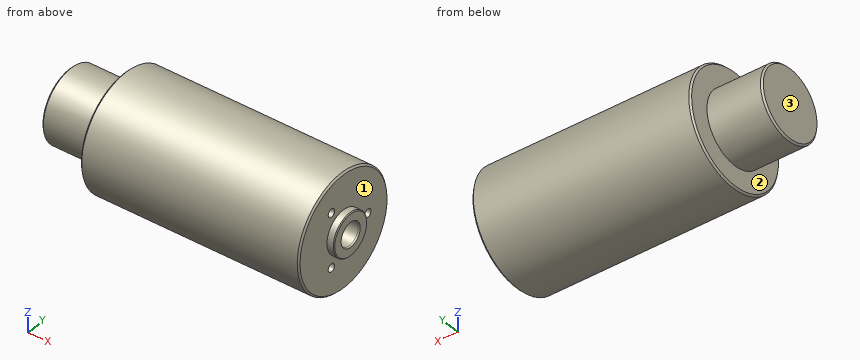
from build123d import *

# Parameters (mm, degrees)
CHANFREIN2_SIZE                   = 0.25
R_P_TITION_CIRCULAIRE1_COUNT      = 3
CHANFREIN3_SIZE                   = 0.5
D_GAGEMENT_POUR_M6_51_D           = 7.1
D_GAGEMENT_POUR_M6_51_DEPTH       = 20
D_GAGEMENT_POUR_M6_51_CSINK_D     = 7.5
D_GAGEMENT_POUR_M6_51_CSINK_ANGLE = 45
D_GAGEMENT_POUR_M6_51_TIP         = 2.133055198


with BuildPart() as part:
    # Esquisse1 → Base-R_volution (revolve)
    with BuildSketch(Plane.XY, mode=Mode.PRIVATE) as base_r_volution_sk:
        Polygon((2.2, 0), (2.2, 6.5), (0, 6.5), (0, 17.5), (-67.500713504, 17.5), (-67.500713504, 11), (-84.500713504, 11), (-84.500713504, 0), align=None)
    revolve(base_r_volution_sk.sketch.rotate(Axis((-71.12515213, 0, 0), (1, 0, 0)), 90), axis=Axis((-71.12515213, 0, 0), (1, 0, 0)))

    # Chanfrein2
    chanfrein2_edges = [part.edges().sort_by_distance(p)[0] for p in [
        (2.2, 0, -6.5),
    ]]
    chamfer(chanfrein2_edges, length=CHANFREIN2_SIZE)

    # Esquisse2 → Trou taraud_ M2.5x0.451 (revolve, cut)
    with BuildSketch(Plane(origin=(0, 9.5, 0), x_dir=(0, 0, -1), z_dir=(0, 1, 0))):
        Polygon((0, 0), (0, 7.365882135), (1.025, 6.75), (1.025, 4.5), (1.25, 4.5), (1.25, 0), align=None)
    trou_taraud_m2_5x0_451 = revolve(axis=Axis((6.35, 9.5, 0), (-1, 0, 0)), mode=Mode.SUBTRACT)

    # R_p_tition circulaire1: Trou taraud_ M2.5x0.451 ×3 about axis
    r_p_tition_circulaire1_axis = Axis((0, 0, 0), (1, 0, 0))
    for i in range(1, R_P_TITION_CIRCULAIRE1_COUNT):
        add(trou_taraud_m2_5x0_451.rotate(r_p_tition_circulaire1_axis, i * 360 / R_P_TITION_CIRCULAIRE1_COUNT), mode=Mode.SUBTRACT)

    # Chanfrein3
    chanfrein3_edges = [part.edges().sort_by_distance(p)[0] for p in [
        (0, 0, -17.5),
        (-67.500713504, 0, -17.5),
        (-84.500713504, 0, -11),
    ]]
    chamfer(chanfrein3_edges, length=CHANFREIN3_SIZE)

    # D_gagement pour M6.51
    with Locations(Plane(origin=(2.2, 0, 0), x_dir=(0, 0, -1), z_dir=(1, 0, 0))):
        with Locations((0, 0)):
            CounterSinkHole(D_GAGEMENT_POUR_M6_51_D / 2, D_GAGEMENT_POUR_M6_51_CSINK_D / 2, depth=D_GAGEMENT_POUR_M6_51_DEPTH, counter_sink_angle=D_GAGEMENT_POUR_M6_51_CSINK_ANGLE)
            with Locations((0, 0, -(D_GAGEMENT_POUR_M6_51_DEPTH + D_GAGEMENT_POUR_M6_51_TIP / 2))):  # 118° drill point
                Cone(0, D_GAGEMENT_POUR_M6_51_D / 2, D_GAGEMENT_POUR_M6_51_TIP, mode=Mode.SUBTRACT)


solid = part.part
Model file for the job. Use its own axes, mm. Face numbers are marked on the shaded views. A direction names the side the tool comes from. Give positions to 0.01 mm unless a question says otherwise; leave off trailing zeros. Loops run counter-clockwise (first coordinate to the right, second up) from the corner with the lowest first, then second, coordinate; pieces in that order, holes last.
Item 1: Drop flat-ended pins along their axis: P1, Ø3, axis at y = 9.5, z = 0, coming from the +X side; P2, Ø1.5, axis at y = 9.5, z = 0, coming from the +X side; P3, Ø1.5, axis at y = -12, z = 6.5, coming from the -X side. Give the stop position or say it passes through.
Check values:
P1: stops at x = 0
P2: stops at x = -6.92
P3: stops at x = -67.5
Item 2: Drill centre lines: line 1 along Y through (x, z) = (-6.5, 0) (3 decimals); line 2 along Y through (x, z) = (-3.25, 0); line 3 along X through (y, z) = (15.5, -3). Where is each one in solid material? Low to high.
Check values:
line 1: y = -17.5 to -3.55, 3.55 to 8.475, 10.525 to 17.5
line 2: y = -17.5 to -3.55, 3.55 to 8.25, 10.75 to 17.5
line 3: x = -67.5 to 0
Item 3: Slice it at B-B (x = -70). Write the cut outline in (y, z).
Check values:
outline: circle Ø22 at (0, 0)
Item 4: Which spindle directions (+Z, -Z, +X, -X, +Y, -Y) get a long thin tool onto all of the face, cutting with end or side? Do the marked faces 1, 2 and 3. Say none if no direction does.
Check values:
face 1: +X
face 2: -X
face 3: +Z, -Z, -X, +Y, -Y
Item 5: Slice it at A-A (x = -58). Write the cut outline in (y, z), plus the area to 3 significant figures.
Check values:
outline: circle Ø35 at (0, 0)
area: 962 mm2
